Input: part model. Units: mm. Frame: model coordinates. A direction names the side the tool comes from. Coordinates: 2 decimals unless noted, no trailing zeros. Loops run counter-clockwise (first coordinate to the right, second up) from the corner with the lowest first, then second, coordinate; pieces in that order, holes last.
Item 1: Pull-direction query (Y, two-part tool) for faces 3 (the cylindrical face through (-123.68, 0.95, 3.13)), 4 (the flat face through (-2, -95, 6.35)); classes: released by +Y, released by -Y, zero draft, split by the parting line, or undercut.
Item 2: Reachability of faces 1 (the flat face through (-2, -95, 0)), 2 (the flat face through (28, -76.835, 3)) from +Z, -Z, +X, -X, +Y, -Y: full face, straight path, thin tool, end or side. Return the list, or none.
Item 3: Section C-C on x = 106. Return loops of the section in (y, z), and give its area (3 significant figures).
Item 4: Contact query for flat-ended pins moving along their axis: P1, Ø3, axis at y = -25, z = 1, coming from the -X side; P2, Ø3, axis at x = 83, z = 5, coming from the +Y side; P3, Ø1, axis at y = 23, z = 3, coming from the +X side. Output: stop coordinate, or through.
Item 5: Section B-B on z = 3.5. Give the number of separate pieces and of enclosed holes in the cut face, and give its area (3 significant figures).
Item 6: Ray query, line 1 along Y through (x, z) = (0, 2) (3 decimals); line 2 along X through (y, z) = (-72.5, 2.25) (3 decimals); line 3 along X through (y, z) = (88.5, 5.75). Return the intervals inside material, ascending.
Item 7: Section A-A on y = 67.5. Return loops of the section in (x, z) (3 decimals).
```python
from build123d import *

# Parameters (mm, degrees)
F0_R     = 146.05
F1_DEPTH = 6.35
F3_D     = 6.35
F4_D     = 9.525
F6_DEPTH = 6.351


with BuildPart() as f1:
    # F0 (on Top) → F1 (new body)
    with BuildSketch(Plane.XY):
        Circle(F0_R)
    extrude(amount=F1_DEPTH)

    # F3 (through all)
    with Locations(Plane.XY.offset(6.35)):
        with Locations((120.65, 0), (0, -120.65), (-120.65, 0), (0, 120.65)):
            Hole(F3_D / 2)

    # F4 (through all)
    with Locations(Plane.XY.offset(6.35)):
        with Locations((-92.586648, -86.929354), (92.586648, 86.929354)):
            Hole(F4_D / 2)

    # F5 (on face) → F6 (cut, through all)
    with BuildSketch(Plane.XY.offset(6.35)):
        with BuildLine():
            Line((76.835, -18.620527), (76.835, 76.835))
            Line((76.835, 76.835), (37.670527, 76.835))
            ThreePointArc((37.670527, 76.835), (28.145527, 86.36), (18.620527, 76.835))
            Line((18.620527, 76.835), (-76.835, 76.835))
            Line((-76.835, 76.835), (-76.835, 37.670527))
            ThreePointArc((-76.835, 37.670527), (-86.36, 28.145527), (-76.835, 18.620527))
            Line((-76.835, 18.620527), (-76.835, -76.835))
            Line((-76.835, -76.835), (-37.670527, -76.835))
            ThreePointArc((-37.670527, -76.835), (-28.145527, -86.36), (-18.620527, -76.835))
            Line((-18.620527, -76.835), (76.835, -76.835))
            Line((76.835, -76.835), (76.835, -37.670527))
            ThreePointArc((76.835, -37.670527), (86.36, -28.145527), (76.835, -18.620527))
        make_face()
    extrude(amount=-F6_DEPTH, mode=Mode.SUBTRACT)


solid = f1.part
```
Results found:
1. face 3: undercut
1. face 4: zero draft
2. face 1: -Z, +X, -X, +Y, -Y
2. face 2: +Z, -Z
3. outline: (-100.47, 0) - (100.47, 0) - (100.47, 6.35) - (-100.47, 6.35) - close
3. area: 1,280 mm2
4. P1: stops at x = -144.15
4. P2: stops at y = 121.2
4. P3: stops at x = 144.31
5. separate pieces: 1
5. enclosed holes: 7
5. area: 42,600 mm2
6. line 1: y = -146.05 to -123.825, -117.475 to -76.835, 76.835 to 117.475, 123.825 to 146.05
6. line 2: x = -126.785 to -76.835, 76.835 to 126.785
6. line 3: x = -116.18 to 88.09, 97.08 to 116.18
7. outline: (-129.516, 0) - (-76.835, 0) - (-76.835, 6.35) - (-129.516, 6.35) - close; (76.835, 0) - (129.516, 0) - (129.516, 6.35) - (76.835, 6.35) - close
